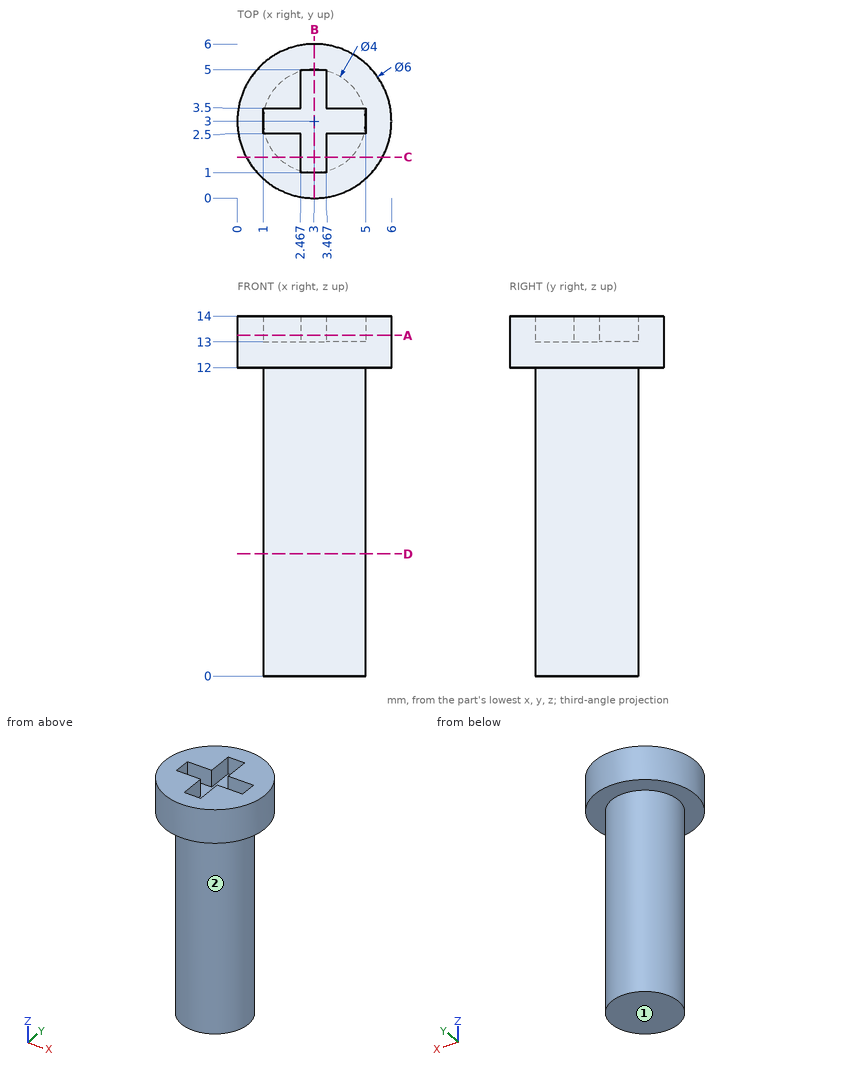
Verification items for this drawing (mm, ordinates from the low corner). A direction names the side the tool comes from. Coordinates: 2 decimals unless noted, no trailing zeros. Loops run counter-clockwise (first coordinate to the right, second up) from the corner with the lowest first, then second, coordinate; pieces in that order, holes last. Notation, with made-up numbers: (36.5, 21) -> (66.5, 21) arc R13 ccw to (66.5, 45) -> close; hole circle Ø4 at (65, 46.5). An arc over 180 degrees is marked (long way). Put each result on its own line as item: value.
1. Section check C-C, the plane y = 1.6. Record the boundary of the cut face in (x, z).
Result set:
outline: (0.35, 12) -> (1.57, 12) -> (1.57, 0) -> (4.43, 0) -> (4.43, 12) -> (5.65, 12) -> (5.65, 14) -> (3.47, 14) -> (3.47, 13) -> (2.47, 13) -> (2.47, 14) -> (0.35, 14) -> close
2. Section check D-D, the plane z = 4.75. Record the boundary of the cut face in (x, y).
Result set:
outline: circle Ø4 at (3, 3)
3. Section check A-A, the plane z = 13.25. Record the boundary of the cut face in (x, y).
Result set:
outline: circle Ø6 at (3, 3); hole (1, 2.5) -> (2.47, 2.5) -> (2.47, 1) -> (3.47, 1) -> (3.47, 2.5) -> (5, 2.5) -> (5, 3.5) -> (3.47, 3.5) -> (3.47, 5) -> (2.47, 5) -> (2.47, 3.5) -> (1, 3.5) -> close
4. Gauge pin test, flat ends, axial feed: P1, Ø3, axis at y = 4, z = 5.5, coming from the -X side; P2, Ø1.1, axis at y = 4, z = 13.5, coming from the +X side; P3, Ø0.8, axis at x = 2.5, z = 13.5, coming from the +Y side; P4, Ø2, axis at x = 1.5, z = 6.5, coming from the -Y side. Record the tip position at first contact, or that the pin passes through.
Result set:
P1: stops at x = 1
P2: stops at x = 5.97
P3: stops at y = 6
P4: stops at y = 1.06
5. Tool access check on the marked faces 1 and 2. Record the directions out of +Z, -Z, +X, -X, +Y, -Y that give a thin tool (end or side, any length) a straight path to the whole face; none if there is none.
Result set:
face 1: -Z, +X, -X, +Y, -Y
face 2: -Z
6. Section check B-B, the plane x = 3. Record the boundary of the cut face in (y, z), then the cut area to 3 significant figures.
Result set:
outline: (0, 12) -> (1, 12) -> (1, 0) -> (5, 0) -> (5, 12) -> (6, 12) -> (6, 14) -> (5, 14) -> (5, 13) -> (1, 13) -> (1, 14) -> (0, 14) -> close
area: 56.0 mm^2
7. Thickness scan on line 1 (Z direction, x = 4.95, y = 2.75); line 2 (Z direction, x = 2.05, y = 4.8); line 3 (X direction, y = 2.9, z = 7). Record the ranges inside material, lowest first.
Result set:
line 1: z = 0 to 13
line 2: z = 12 to 14
line 3: x = 1 to 5
